The listing builds one solid part. Answer for the finished solid, in the listing's coordinates (mm). A direction names the side the tool comes from. Give positions to 0.01 mm unless a question says otherwise; leave off trailing zeros. Loops run counter-clockwise (first coordinate to the right, second up) from the corner with the lowest first, then second, coordinate; pieces in that order, holes last. Notation, with made-up numbers: (-11, 68) -> (43, 68) arc R24 cw to (43, 107) -> close; hole circle Ø6 at (-17.5, 44.5). An arc over 180 degrees is marked (long way). One line per question, with ' | ' between items. Start each with the question number.
from build123d import *

# Parameters (mm, degrees)
SKETCH1_W               = 35.5
SKETCH1_H               = 44.45
BOSS_EXTRUDE1_DEPTH     = 2
SKETCH2_R               = 1.75
CUT_EXTRUDE1_DEPTH      = 29.513385015
SKETCH3_W               = 7
SKETCH3_H               = 26.45
CUT_EXTRUDE2_DEPTH      = 29.513385015
FILLET1_R               = 2
SKETCH4_W               = 2
SKETCH4_H               = 30
BOSS_EXTRUDE3_DEPTH     = 15
FILLET2_R               = 15
SKETCH5_R               = 1.75
CUT_EXTRUDE3_DEPTH      = 39.710633229
CIRPATTERN1_COUNT       = 7
CIRPATTERN1_ANGLE       = 150
MIRROR1_COPY_1_SKETCH_R = 1.75
MIRROR1_COPY_1_DEPTH    = 39.710633229
MIRROR1_COPY_2_SKETCH_R = 1.75
MIRROR1_COPY_2_DEPTH    = 39.710633229
MIRROR1_COPY_3_SKETCH_R = 1.75
MIRROR1_COPY_3_DEPTH    = 39.710633229
MIRROR1_COPY_4_SKETCH_R = 1.75
MIRROR1_COPY_4_DEPTH    = 39.710633229
MIRROR1_COPY_5_SKETCH_R = 1.75
MIRROR1_COPY_5_DEPTH    = 39.710633229
MIRROR1_COPY_6_SKETCH_R = 1.75
MIRROR1_COPY_6_DEPTH    = 39.710633229
FILLET2_OF_MIRROR1_R    = 15


with BuildPart() as part:
    # Sketch1 → Boss-Extrude1 (new body)
    with BuildSketch(Plane(origin=(0, 0, 0), x_dir=(1, 0, 0), z_dir=(0, 1, 0))):
        Rectangle(SKETCH1_W, SKETCH1_H)
    extrude(amount=BOSS_EXTRUDE1_DEPTH)

    # Sketch2 → Cut-Extrude1 (cut, through all)
    with BuildSketch(Plane(origin=(0, 2, 0), x_dir=(1, 0, 0), z_dir=(0, 1, 0))):
        with Locations(Location((-14.5, 18.725, 0), (0, 0, 270))):
            Circle(SKETCH2_R)
        with Locations(Location((14.5, 18.725, 0), (0, 0, 270))):
            Circle(SKETCH2_R)
    extrude(amount=-CUT_EXTRUDE1_DEPTH, mode=Mode.SUBTRACT)

    # Sketch3 → Cut-Extrude2 (cut, through all)
    with BuildSketch(Plane(origin=(0, 2, 0), x_dir=(1, 0, 0), z_dir=(0, 1, 0))):
        with Locations((-14.25, -9)):
            Rectangle(SKETCH3_W, SKETCH3_H)
        with Locations((14.25, -9)):
            Rectangle(SKETCH3_W, SKETCH3_H)
    extrude(amount=-CUT_EXTRUDE2_DEPTH, mode=Mode.SUBTRACT)

    # Fillet1
    fillet1_edges = [part.edges().sort_by_distance(p)[0] for p in [
        (-17.75, 1, -4.225),
        (-10.75, 1, -4.225),
        (-10.75, 1, 22.225),
        (17.75, 1, -4.225),
        (10.75, 1, 22.225),
        (10.75, 1, -4.225),
        (-17.75, 1, -22.225),
        (17.75, 1, -22.225),
    ]]
    fillet(fillet1_edges, radius=FILLET1_R)

    # Sketch4 → Boss-Extrude3 (add)
    with BuildSketch(Plane(origin=(0, 2, 0), x_dir=(1, 0, 0), z_dir=(0, 1, 0))):
        with Locations((-8, 0)):
            Rectangle(SKETCH4_W, SKETCH4_H)
    boss_extrude3 = extrude(amount=BOSS_EXTRUDE3_DEPTH)

    # Fillet2
    fillet2_edges = [part.edges().sort_by_distance(p)[0] for p in [
        (-8, 17, 15),
        (-8, 17, -15),
    ]]
    fillet(fillet2_edges, radius=FILLET2_R - 0.0001)  # a hair under: the kernel refuses the full size

    # Sketch5 → Cut-Extrude3 (cut, through all)
    with BuildSketch(Plane.ZY.offset(9)):
        with Locations((10.428326807, 5.5)):
            Circle(SKETCH5_R)
    cut_extrude3 = extrude(amount=-CUT_EXTRUDE3_DEPTH, mode=Mode.SUBTRACT)

    # CirPattern1: Cut-Extrude3 ×7 about axis
    cirpattern1_axis = Axis((0, 2, 0), (-1, 0, 0))
    for i in range(1, CIRPATTERN1_COUNT):
        add(cut_extrude3.rotate(cirpattern1_axis, i * CIRPATTERN1_ANGLE / (CIRPATTERN1_COUNT - 1)), mode=Mode.SUBTRACT)

    # Mirror1: Boss-Extrude3, Cut-Extrude3 across plane
    add(boss_extrude3.mirror(Plane(origin=(0, 0, 0), x_dir=(0, 0, 1), z_dir=(1, 0, 0))))
    add(cut_extrude3.mirror(Plane(origin=(0, 0, 0), x_dir=(0, 0, 1), z_dir=(1, 0, 0))), mode=Mode.SUBTRACT)

    # Mirror1 copy 1 sketch → Mirror1 copy 1 (cut, through all)
    with BuildSketch(Plane(origin=(9, 0.187384426, 0.845236523), x_dir=(0, 0.42261826174070033, 0.9063077870366495), z_dir=(1, 0, 0))):
        with Locations((10.428326807, -5.5)):
            Circle(MIRROR1_COPY_1_SKETCH_R)
    extrude(amount=-MIRROR1_COPY_1_DEPTH, mode=Mode.SUBTRACT)

    # Mirror1 copy 2 sketch → Mirror1 copy 2 (cut, through all)
    with BuildSketch(Plane(origin=(9, 0.714424781, 1.532088886), x_dir=(0, 0.7660444431189793, 0.6427876096865378), z_dir=(1, 0, 0))):
        with Locations((10.428326807, -5.5)):
            Circle(MIRROR1_COPY_2_SKETCH_R)
    extrude(amount=-MIRROR1_COPY_2_DEPTH, mode=Mode.SUBTRACT)

    # Mirror1 copy 3 sketch → Mirror1 copy 3 (cut, through all)
    with BuildSketch(Plane(origin=(9, 1.48236191, 1.931851653), x_dir=(0, 0.9659258262890691, 0.25881904510251796), z_dir=(1, 0, 0))):
        with Locations((10.428326807, -5.5)):
            Circle(MIRROR1_COPY_3_SKETCH_R)
    extrude(amount=-MIRROR1_COPY_3_DEPTH, mode=Mode.SUBTRACT)

    # Mirror1 copy 4 sketch → Mirror1 copy 4 (cut, through all)
    with BuildSketch(Plane(origin=(9, 2.347296355, 1.969615506), x_dir=(0, 0.9848077530122074, -0.17364817766693424), z_dir=(1, 0, 0))):
        with Locations((10.428326807, -5.5)):
            Circle(MIRROR1_COPY_4_SKETCH_R)
    extrude(amount=-MIRROR1_COPY_4_DEPTH, mode=Mode.SUBTRACT)

    # Mirror1 copy 5 sketch → Mirror1 copy 5 (cut, through all)
    with BuildSketch(Plane(origin=(9, 3.147152873, 1.638304089), x_dir=(0, 0.8191520442889889, -0.5735764363510502), z_dir=(1, 0, 0))):
        with Locations((10.428326807, -5.5)):
            Circle(MIRROR1_COPY_5_SKETCH_R)
    extrude(amount=-MIRROR1_COPY_5_DEPTH, mode=Mode.SUBTRACT)

    # Mirror1 copy 6 sketch → Mirror1 copy 6 (cut, through all)
    with BuildSketch(Plane(origin=(9, 3.732050808, 1), x_dir=(0, 0.49999999999999495, -0.8660254037844416), z_dir=(1, 0, 0))):
        with Locations((10.428326807, -5.5)):
            Circle(MIRROR1_COPY_6_SKETCH_R)
    extrude(amount=-MIRROR1_COPY_6_DEPTH, mode=Mode.SUBTRACT)

    # Fillet2 of Mirror1
    fillet2_of_mirror1_edges = [part.edges().sort_by_distance(p)[0] for p in [
        (8, 17, 15),
        (8, 17, -15),
    ]]
    fillet(fillet2_of_mirror1_edges, radius=FILLET2_OF_MIRROR1_R - 0.0001)  # a hair under: the kernel refuses the full size


solid = part.part
1. The part is cut by section B-B (y = 12.75). Count the separate pieces of the cut face and the enclosed holes in it, plus the area to 3 significant figures.
2. The part is cut by section C-C (z = 7). Write down the section's boundary in (x, y), plus the area to 3 significant figures.
3. Each of these flat-tipped pins is pushed along its axis until it touches: pin 1 Ø2 at (x, z) = (-2.5, -13) entering from +Y; pin 2 Ø4.5 at (y, z) = (12.24, 4.02) entering from +X; pin 3 Ø4.5 at (y, z) = (8.53, -8.85) entering from -X; pin 4 Ø2 at (y, z) = (12.98, -0.68) entering from +X. Where does it stop, or does it pass through?
4. For faces 1 (the flat face through (-9, 8, 0)), 2 (the cylindrical face through (-8.01, 9.66, 9.72)), determine the directions among +Z, -Z, +X, -X, +Y, -Y from which every point of the face is accessible in a straight line to the end or side of a thin tool.
5. Determine the mould class of faces 3 (the cylindrical face through (8.014, 10.204, -9.375)), 4 (the cylindrical face through (7.99, 12.49, -10.72)), 5 (the flat face through (9, 8, 0)) for opening direction Z: released by +Z, released by -Z, zero draft, split by the parting line, or undercut.
6. The part is cut by section A-A (x = -14.5). Write down the section's boundary in (y, z) (3 decimals).
7. Straight lines are drawn through the part: L1, parallel to X at y = 4, z = -8.5; L2, parallel to Y at x = -1, z = -2.5; L3, parallel to X at y = 1.75, z = -6. For each, find the intervals that lie inside material, in ascending order.
Check sheet entries:
1) separate pieces: 8 | enclosed holes: 0 | area: 45.5 mm^2
2) outline: (-10.75, 0) -> (10.75, 0) -> (10.75, 2) -> (9, 2) -> (9, 8.12) -> (7, 8.12) -> (7, 2) -> (-7, 2) -> (-7, 8.12) -> (-9, 8.12) -> (-9, 2) -> (-10.75, 2) -> close; (-9, 11.03) -> (-7, 11.03) -> (-7, 15.27) -> (-9, 15.27) -> close; (7, 11.03) -> (9, 11.03) -> (9, 15.27) -> (7, 15.27) -> close | area: 84.4 mm^2
3) pin 1: stops at y = 2 | pin 2: stops at x = 9 | pin 3: stops at x = -9 | pin 4: passes through
4) face 1: +Z, -Z, -X, +Y | face 2: +X, -X
5) face 3: undercut | face 4: released by -Z | face 5: zero draft
6) outline: (0, -22.225) -> (2, -22.225) -> (2, -20.475) -> (0, -20.475) -> close; (0, -16.975) -> (2, -16.975) -> (2, -4.225) -> (0, -4.225) -> close
7) L1: x = -9 to -7, 7 to 9 | L2: y = 0 to 2 | L3: x = -17.74 to 17.74
